```python
from build123d import *

# Parameters (mm, degrees)
SKETCH1_R           = 2.5
BOSS_EXTRUDE1_DEPTH = 6


with BuildPart() as part:
    # Sketch1 → Boss-Extrude1 (new body)
    with BuildSketch(Plane(origin=(0, 0, 0), x_dir=(0, 0, -1), z_dir=(1, 0, 0))):
        Polygon((0, 0), (400, 0), (400, 400), (200, 400), (0, 60), align=None)
        with Locations((30, 42)):
            Circle(SKETCH1_R, mode=Mode.SUBTRACT)
        with Locations(Location((30, 18, 0), (0, 0, 180))):
            Circle(SKETCH1_R, mode=Mode.SUBTRACT)
        with Locations((370, 18)):
            Circle(SKETCH1_R, mode=Mode.SUBTRACT)
        with Locations(Location((370, 42, 0), (0, 0, 180))):
            Circle(SKETCH1_R, mode=Mode.SUBTRACT)
        with Locations((310, 350)):
            Circle(SKETCH1_R, mode=Mode.SUBTRACT)
        with Locations((310, 250)):
            Circle(SKETCH1_R, mode=Mode.SUBTRACT)
    extrude(amount=BOSS_EXTRUDE1_DEPTH)


solid = part.part
```
Geometry: final body of the model. Coordinates: model frame, mm. Round coordinates to 2 decimals unless told otherwise and drop trailing zeros. Order: outer loops, then holes, each group sorted by start corner. A loop starts at its lowest first (then second) coordinate and runs counter-clockwise, first axis right, second up. Notation, with made-up numbers: M -16.5,46 L 40.5,46 A17 ccw 40.5,71 Z; hole C 70,17 d3. An arc over 180 degrees is marked long. One line per item, written item: value.
(1) Pin query (flat end, axial travel): P1, Ø8, axis at y = 18, z = -30, coming from the -X side; P2, Ø2, axis at x = 2.5, y = 241, coming from the +Z side; P3, Ø1, axis at x = 1, y = 346, coming from the +Z side. Return the tip coordinate at first contact, or that it passes through.
Result sheet:
P1: x = 0
P2: z = -105.88
P3: z = -167.94
(2) Cut plane C-C (y = 370.5). Return the cut outline in (x, z), and give its area (3 significant figures).
Result sheet:
outline: M 0,-400 L 6,-400 L 6,-182.65 L 0,-182.65 Z
area: 1,300 mm2
(3) Cut plane B-B (z = -144.5). Return the cut outline in (x, y).
Result sheet:
outline: M 0,0 L 6,0 L 6,305.65 L 0,305.65 Z
(4) Line query: probe 1 along Y at (x, z) = (3.45, -370); probe 2 along Y at (x, z) = (2, -310); probe 3 along Z at (x, y) = (3.05, 250). Output: solid intervals per line, ascending. Write a range as [from, to].
Result sheet:
probe 1: [0, 15.5], [20.5, 39.5], [44.5, 400]
probe 2: [0, 247.5], [252.5, 347.5], [352.5, 400]
probe 3: [-400, -312.5], [-307.5, -111.76]
(5) Cut plane A-A (x = 4.95). Return the cut outline in (y, z).
Result sheet:
outline: M 0,-400 L 400,-400 L 400,-200 L 60,0 L 0,0 Z; hole C 18,-370 d5; hole C 18,-30 d5; hole C 42,-370 d5; hole C 42,-30 d5; hole C 250,-310 d5; hole C 350,-310 d5
